Check sheet for the modelled part. Datum: model origin and axes. Units: mm. Face numbers are marked on the shaded views. A direction names the side the tool comes from. Round coordinates to 2 decimals unless told otherwise and drop trailing zeros. Loops run counter-clockwise (first coordinate to the right, second up) from the corner with the lowest first, then second, coordinate; pieces in that order, holes last. Notation, with made-up numbers: (-38, -12.5) -> (-27, -12.5) arc R18 cw to (-27, 15.5) -> close; hole circle Ø9 at (42.25, 24). An arc over 180 degrees is marked (long way). One line per question, with ' | ' between items.
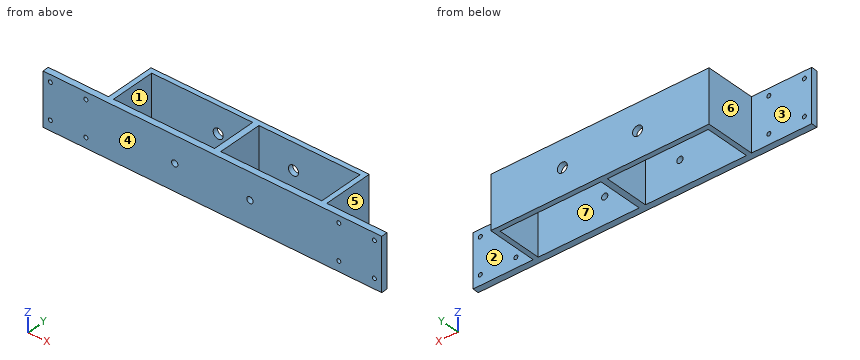
```python
from build123d import *

# Parameters (mm, degrees)
SKETCH1_W           = 171.45
SKETCH1_H           = 26.67
SKETCH1_R           = 1.016
BOSS_EXTRUDE1_DEPTH = 3.175
SKETCH2_W           = 2.54
SKETCH2_H           = 26.67
BOSS_EXTRUDE2_DEPTH = 22.86
SKETCH3_W           = 26.67
SKETCH3_H           = 2.54
BOSS_EXTRUDE3_DEPTH = 110.49
SKETCH4_R           = 1.5875
CUT_EXTRUDE1_DEPTH  = 3.175
SKETCH5_R           = 2.54
CUT_EXTRUDE2_DEPTH  = 2.54
SKETCH6_W           = 3.175
SKETCH6_H           = 26.67
BOSS_EXTRUDE4_DEPTH = 22.86


with BuildPart() as part:
    # Sketch1 → Boss-Extrude1 (new body)
    with BuildSketch(Plane(origin=(0, 0, 0), x_dir=(1, 0, 0), z_dir=(0, 1, 0))):
        with Locations((0, 13.335)):
            Rectangle(SKETCH1_W, SKETCH1_H)
        with Locations(Location((64.025, 21.59, 0), (0, 0, 270))):
            Circle(SKETCH1_R, mode=Mode.SUBTRACT)
        with Locations(Location((82.025, 21.59, 0), (0, 0, 270))):
            Circle(SKETCH1_R, mode=Mode.SUBTRACT)
        with Locations(Location((64.025, 3.59, 0), (0, 0, 270))):
            Circle(SKETCH1_R, mode=Mode.SUBTRACT)
        with Locations(Location((82.025, 3.59, 0), (0, 0, 270))):
            Circle(SKETCH1_R, mode=Mode.SUBTRACT)
        with Locations(Location((-82.025, 3.59, 0), (0, 0, 90))):
            Circle(SKETCH1_R, mode=Mode.SUBTRACT)
        with Locations(Location((-64.025, 3.59, 0), (0, 0, 90))):
            Circle(SKETCH1_R, mode=Mode.SUBTRACT)
        with Locations(Location((-82.025, 21.59, 0), (0, 0, 90))):
            Circle(SKETCH1_R, mode=Mode.SUBTRACT)
        with Locations(Location((-64.025, 21.59, 0), (0, 0, 90))):
            Circle(SKETCH1_R, mode=Mode.SUBTRACT)
    extrude(amount=BOSS_EXTRUDE1_DEPTH)

    # Sketch2 → Boss-Extrude2 (add)
    with BuildSketch(Plane(origin=(0, 3.175, 0), x_dir=(1, 0, 0), z_dir=(0, 1, 0))):
        with Locations((-53.975, 13.335)):
            Rectangle(SKETCH2_W, SKETCH2_H)
    boss_extrude2 = extrude(amount=BOSS_EXTRUDE2_DEPTH)

    # Mirror1: Boss-Extrude2 across plane
    add(boss_extrude2.mirror(Plane(origin=(0, 0, 0), x_dir=(0, 0, 1), z_dir=(1, 0, 0))))

    # Sketch3 → Boss-Extrude3 (add)
    with BuildSketch(Plane.ZY.offset(55.245)):
        with Locations((-13.335, 27.305)):
            Rectangle(SKETCH3_W, SKETCH3_H)
    extrude(amount=-BOSS_EXTRUDE3_DEPTH)

    # Sketch4 → Cut-Extrude1 (cut)
    with BuildSketch(Plane(origin=(0, 3.175, 0), x_dir=(1, 0, 0), z_dir=(0, 1, 0))):
        with Locations(Location((-19.05, 13.335, 0), (0, 0, 270))):
            Circle(SKETCH4_R)
        with Locations(Location((19.05, 13.335, 0), (0, 0, 270))):
            Circle(SKETCH4_R)
    extrude(amount=-CUT_EXTRUDE1_DEPTH, mode=Mode.SUBTRACT)

    # Sketch5 → Cut-Extrude2 (cut)
    with BuildSketch(Plane(origin=(0, 28.575, 0), x_dir=(1, 0, 0), z_dir=(0, 1, 0))):
        with Locations(Location((-19.05, 13.335, 0), (0, 0, 270))):
            Circle(SKETCH5_R)
        with Locations(Location((19.05, 13.335, 0), (0, 0, 270))):
            Circle(SKETCH5_R)
    extrude(amount=-CUT_EXTRUDE2_DEPTH, mode=Mode.SUBTRACT)

    # Sketch6 → Boss-Extrude4 (add)
    with BuildSketch(Plane(origin=(0, 3.175, 0), x_dir=(1, 0, 0), z_dir=(0, 1, 0))):
        with Locations((0, 13.335)):
            Rectangle(SKETCH6_W, SKETCH6_H)
    extrude(amount=BOSS_EXTRUDE4_DEPTH)


solid = part.part
```
(1) Scan lines: probe 1 along X at (y, z) = (15.5, -18.25) (1 decimal); probe 2 along X at (y, z) = (1.6, -3.59) (3 decimals); probe 3 along Y at (x, z) = (4, -15) (3 decimals). Record each from-to range of solid material in increasing order.
Answer:
probe 1: x = -55.2 to -52.7, -1.6 to 1.6, 52.7 to 55.2 | probe 2: x = -85.725 to -83.041, -81.009 to -65.041, -63.009 to 63.009, 65.041 to 81.009, 83.041 to 85.725 | probe 3: y = 0 to 3.175, 26.035 to 28.575
(2) Set-up check for the marked faces 1, 2 and 3: record each of +Z, -Z, +X, -X, +Y, -Y from which the full face is reachable in a straight line by a thin tool's end or side.
Answer:
face 1: +Z, -Z | face 2: +Z, -Z, +X, +Y | face 3: +Z, -Z, -X, +Y
(3) Sectioned sample at D-D, the plane x = 19.05. Record the cut outline in (y, z) (1 decimal).
Answer:
outline: (0, -26.7) -> (3.2, -26.7) -> (3.2, -14.9) -> (0, -14.9) -> close; (0, -11.7) -> (3.2, -11.7) -> (3.2, 0) -> (0, 0) -> close; (26, -26.7) -> (28.6, -26.7) -> (28.6, -15.9) -> (26, -15.9) -> close; (26, -10.8) -> (28.6, -10.8) -> (28.6, 0) -> (26, 0) -> close
(4) Sectioned sample at B-B, the plane x = -41.5. Record the cut outline in (y, z) (3 decimals), and give its area (3 significant figures).
Answer:
outline: (0, -26.67) -> (3.175, -26.67) -> (3.175, 0) -> (0, 0) -> close; (26.035, -26.67) -> (28.575, -26.67) -> (28.575, 0) -> (26.035, 0) -> close | area: 152 mm2
(5) Sectioned sample at C-C, the plane z = -18.75. Record the cut outline in (x, y) (1 decimal).
Answer:
outline: (-85.7, 0) -> (85.7, 0) -> (85.7, 3.2) -> (55.2, 3.2) -> (55.2, 28.6) -> (-55.2, 28.6) -> (-55.2, 3.2) -> (-85.7, 3.2) -> close; hole (-52.7, 3.2) -> (-1.6, 3.2) -> (-1.6, 26) -> (-52.7, 26) -> close; hole (1.6, 3.2) -> (52.7, 3.2) -> (52.7, 26) -> (1.6, 26) -> close
(6) Go/stop test with flat-tipped pins: pin 1 (7 mm diameter, centred on y = 13.5, z = -14, fed in from -X) (3 decimals); pin 2 (13.5 mm diameter, centred on x = 67, z = -17.5, fed in from +Y) (3 decimals); pin 3 (12 mm diameter, centred on y = 13.5, z = -16.5, fed in from +X) (3 decimals). Record where each tip stops, or that it passes through.
Answer:
pin 1: stops at x = -55.245 | pin 2: stops at y = 3.175 | pin 3: stops at x = 55.245
(7) Sectioned sample at A-A, the plane y = 8.25. Record the cut outline in (x, z) (1 decimal), and give its area (3 significant figures).
Answer:
outline: (-55.2, -26.7) -> (-52.7, -26.7) -> (-52.7, 0) -> (-55.2, 0) -> close; (-1.6, -26.7) -> (1.6, -26.7) -> (1.6, 0) -> (-1.6, 0) -> close; (52.7, -26.7) -> (55.2, -26.7) -> (55.2, 0) -> (52.7, 0) -> close | area: 220 mm2
(8) Mould release check, pull along X, two halves, no side actions. Record for the marked faces 4, 5, 6 and 7: +X half, -X half, draft (parallel to the pull), parting line (faces both ways), or undercut.
Answer:
face 4: draft | face 5: +X half | face 6: -X half | face 7: undercut
